Input: part model. Units: mm. Frame: model coordinates. Coordinates: 2 decimals unless noted, no trailing zeros. Order: outer loops, then holes, each group sorted by start corner. A loop starts at its lowest first (then second) coordinate and runs counter-clockwise, first axis right, second up. Notation, with made-up numbers: (59.25, -6) -> (71.25, -6) arc R18 ccw to (71.25, 23) -> close; hole circle Ø8 at (-37.75, -15.75). An arc over 180 degrees is marked (long way). Write each question's results on one line, items separated by ' | '.
```python
from build123d import *

# Parameters (mm, degrees)
SKETCH_R   = 210
SKETCH_R_2 = 32
SKETCH_R_3 = 2.5
SKETCH_W   = 22
SKETCH_H   = 100
SKETCH_W_2 = 200
SKETCH_H_2 = 250
PAD_DEPTH  = 1.5


with BuildPart() as part:
    # Sketch → Pad (new body, symmetric)
    with BuildSketch(Plane.XY):
        Circle(SKETCH_R)
        with Locations((0, 170)):
            Circle(SKETCH_R_2, mode=Mode.SUBTRACT)
        with Locations((0, -170)):
            Circle(SKETCH_R_2, mode=Mode.SUBTRACT)
        with Locations((-141, 33.5)):
            Circle(SKETCH_R_3, mode=Mode.SUBTRACT)
        with Locations((-141, -33.5)):
            Circle(SKETCH_R_3, mode=Mode.SUBTRACT)
        with Locations((-115, 33.5)):
            Circle(SKETCH_R_3, mode=Mode.SUBTRACT)
        with Locations((-115, -33.5)):
            Circle(SKETCH_R_3, mode=Mode.SUBTRACT)
        with Locations((115, 33.5)):
            Circle(SKETCH_R_3, mode=Mode.SUBTRACT)
        with Locations((115, -33.5)):
            Circle(SKETCH_R_3, mode=Mode.SUBTRACT)
        with Locations((145, 33.5)):
            Circle(SKETCH_R_3, mode=Mode.SUBTRACT)
        with Locations((145, -33.5)):
            Circle(SKETCH_R_3, mode=Mode.SUBTRACT)
        with Locations((-90, 172.29129)):
            Circle(SKETCH_R_3, mode=Mode.SUBTRACT)
        with Locations((90, 172.29129)):
            Circle(SKETCH_R_3, mode=Mode.SUBTRACT)
        with Locations((-30, 200)):
            Circle(SKETCH_R_3, mode=Mode.SUBTRACT)
        with Locations((30, 200)):
            Circle(SKETCH_R_3, mode=Mode.SUBTRACT)
        with Locations((-30, 140)):
            Circle(SKETCH_R_3, mode=Mode.SUBTRACT)
        with Locations((30, 140)):
            Circle(SKETCH_R_3, mode=Mode.SUBTRACT)
        with Locations((-30, -140)):
            Circle(SKETCH_R_3, mode=Mode.SUBTRACT)
        with Locations((30, -140)):
            Circle(SKETCH_R_3, mode=Mode.SUBTRACT)
        with Locations((-30, -200)):
            Circle(SKETCH_R_3, mode=Mode.SUBTRACT)
        with Locations((30, -200)):
            Circle(SKETCH_R_3, mode=Mode.SUBTRACT)
        with Locations((-172, 0)):
            Rectangle(SKETCH_W, SKETCH_H, mode=Mode.SUBTRACT)
        with Locations((172, 0)):
            Rectangle(SKETCH_W, SKETCH_H, mode=Mode.SUBTRACT)
        Rectangle(SKETCH_W_2, SKETCH_H_2, mode=Mode.SUBTRACT)
    extrude(amount=PAD_DEPTH, both=True)


solid = part.part
```
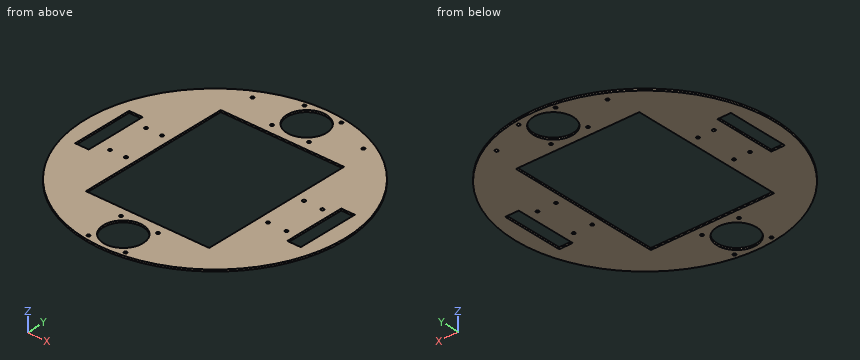
(1) Cut plane A-A, the plane y = 0. Return loops of the section in (x, z), plus the area to 3 significant figures.
Return value:
outline: (-210, -1.5) -> (-183, -1.5) -> (-183, 1.5) -> (-210, 1.5) -> close; (-161, -1.5) -> (-100, -1.5) -> (-100, 1.5) -> (-161, 1.5) -> close; (100, -1.5) -> (161, -1.5) -> (161, 1.5) -> (100, 1.5) -> close; (183, -1.5) -> (210, -1.5) -> (210, 1.5) -> (183, 1.5) -> close | area: 528 mm2
(2) Line query: line 1 along X through (y, z) = (-5, 0.2); line 2 along X through (y, z) = (47.5, 0.25); line 3 along Y through (x, z) = (-115, 0.8). Output: solid intervals per line, ascending. Write a range as from..to.
Return value:
line 1: -209.94..-183, -161..-100, 100..161, 183..209.94 | line 2: -204.56..-183, -161..-100, 100..161, 183..204.56 | line 3: -175.71..-36, -31..31, 36..175.71
(3) Cut plane B-B, the plane y = -170. Return loops of the section in (x, z), plus the area to 3 significant figures.
Return value:
outline: (-123.29, -1.5) -> (-32, -1.5) -> (-32, 1.5) -> (-123.29, 1.5) -> close; (32, -1.5) -> (123.29, -1.5) -> (123.29, 1.5) -> (32, 1.5) -> close | area: 548 mm2
(4) Cut plane D-D, the plane z = 0.8. Count the separate pieces of the cut face and the enclosed holes in it, plus the area to 3 significant figures.
Return value:
separate pieces: 1 | enclosed holes: 23 | area: 77,400 mm2
(5) Pin query (flat end, axial travel): P1, Ø4, axis at x = -30, y = -200, coming from the -Z side; P2, Ø1, axis at x = -81, z = 0.5, coming from the +Y side; P3, Ø6, axis at x = -141, y = 33.5, coming from the -Z side; P4, Ø0.9, axis at x = -173, z = -0.5, coming from the +Y side. Return the tip coordinate at first contact, or that it passes through.
Return value:
P1: through | P2: y = 193.96 | P3: z = -1.5 | P4: y = 119.69
(6) Cut plane C-C, the plane x = 49. Return loops of the section in (y, z), plus the area to 3 significant figures.
Return value:
outline: (-204.2, -1.5) -> (-125, -1.5) -> (-125, 1.5) -> (-204.2, 1.5) -> close; (125, -1.5) -> (204.2, -1.5) -> (204.2, 1.5) -> (125, 1.5) -> close | area: 475 mm2
